Input: dimensioned drawing with shaded views. Units: mm. Origin: part minimum x, y, z. A direction names the side the tool comes from. Round coordinates to 2 decimals unless told otherwise and drop trailing zeros. Loops run counter-clockwise (first coordinate to the right, second up) from the corner with the lowest first, then second, coordinate; pieces in that order, holes last. Notation, with made-up numbers: (-16.5, -17.75) - (12.5, -17.75) arc R20 cw to (12.5, 18.25) - close; hole circle Ø9 at (65.25, 40). An arc over 180 degrees is marked (long way). Answer as a JSON object with one key per item and string values. Group by question number.
Item 1: Section B-B (x = 13.5). Return the cut outline in (y, z).
Item 2: Reachability of the marked faces 1, 2 and 3 from +Z, -Z, +X, -X, +Y, -Y: full face, straight path, thin tool, end or side. Return the list, or none.
Item 3: Section C-C (z = 10.75). Return the cut outline in (x, y).
Item 4: Line query: line 1 (X direction, y = 28.5, z = 4.25); line 2 (Z direction, x = 20, y = 20); line 3 (Y direction, x = 6, z = 7.5). Output: solid intervals per line, ascending.
Item 5: Section A-A (y = 24.5). Return the cut outline in (x, z).
Item 6: Section D-D (x = 17.25). Return the cut outline in (y, z).
Item 7: First-contact query: pin 1 (2 mm diameter, centred on x = 19.5, y = 3.5, fed in from -Z); pin 2 (2 mm diameter, centred on y = 23, z = 9.5, fed in from -X); pin 3 (0.8 mm diameter, centred on x = 6, y = 33.5, fed in from +Z). Flat tips, straight axial feed; report the tip coordinate or a pass-through.
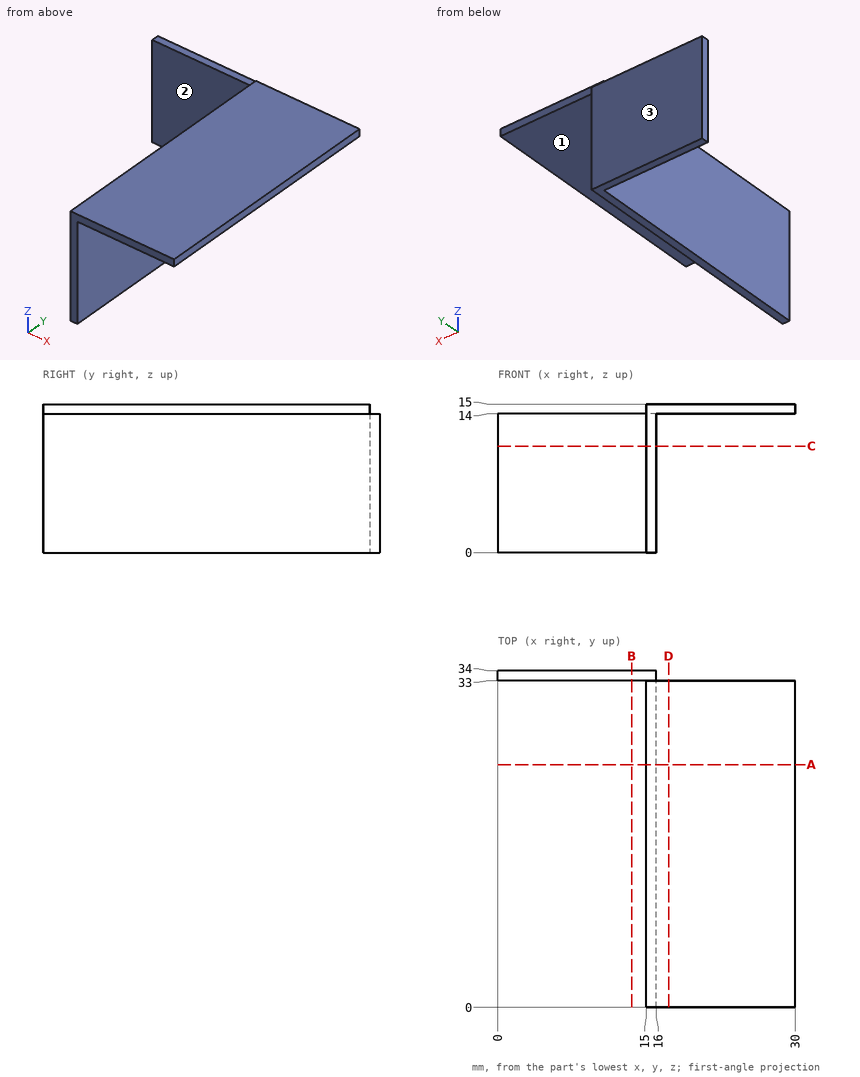
Values:
{
 "1": {"outline": "(33, 0) - (34, 0) - (34, 14) - (33, 14) - close"},
 "2": {"face 1": "-Z, +X, +Y, -Y", "face 2": "+Z, -Z, -X, -Y", "face 3": "+Z, -Z, +X, -X, +Y"},
 "3": {"outline": "(0, 33) - (15, 33) - (15, 0) - (16, 0) - (16, 34) - (0, 34) - close"},
 "4": {"line 1": "x = 15 to 16", "line 2": "z = 14 to 15", "line 3": "y = 33 to 34"},
 "5": {"outline": "(15, 0) - (16, 0) - (16, 14) - (30, 14) - (30, 15) - (15, 15) - close"},
 "6": {"outline": "(0, 14) - (33, 14) - (33, 15) - (0, 15) - close"},
 "7": {"pin 1": "stops at z = 14", "pin 2": "stops at x = 15", "pin 3": "stops at z = 14"}
}
